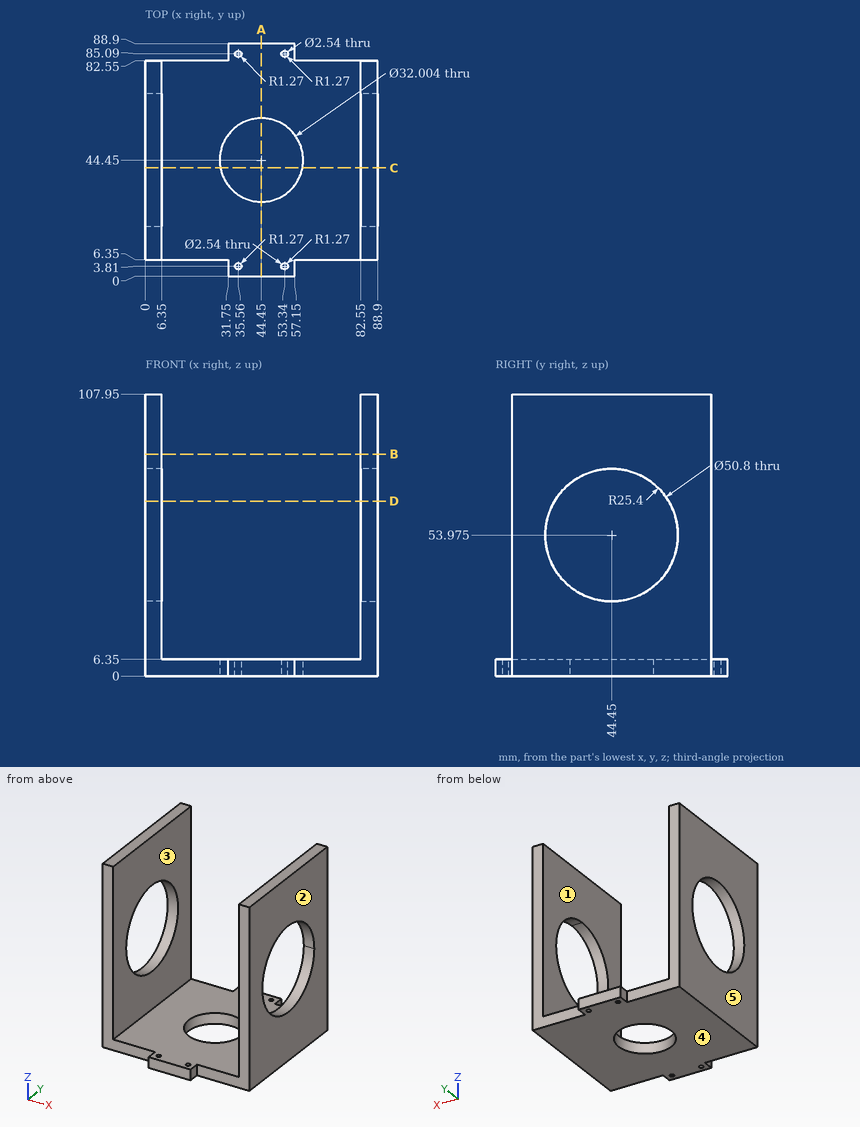
Study the drawing (mm; zero at the part's minimum x, y, z) and answer. A direction names the side the tool comes from. Give positions to 0.01 mm unless a question says otherwise; leave off trailing zeros. Write each loop counter-clockwise with the first axis right and the second up, starting at its lowest first coordinate (ties: lowest second). Pieces come first, ordered by that corner, then holes. Notation, with made-up numbers: (28.25, 79.5) -> (64.25, 79.5) arc R16 ccw to (64.25, 100.5) -> close; hole circle Ø1 at (18, -17). An arc over 180 degrees is marked (long way). Answer in a Markdown table with one row per item.
1) Each of these flat-tipped pins is pushed along its axis until it touches: pin 1 Ø3.5 at (x, y) = (53.34, 85.09) entering from +Z; pin 2 Ø1.9 at (y, z) = (3.5, 4) entering from +X; pin 3 Ø16 at (x, z) = (22, 71.5) entering from +Y; pin 4 Ø1.9 at (y, z) = (4, 3.5) entering from -X. Where does it stop, or does it pass through?
Results list:
| item | result |
|---|---|
| pin 1 | z = 6.35 |
| pin 2 | x = 57.15 |
| pin 3 | through |
| pin 4 | x = 31.75 |
2) Section A-A on x = 44.45 is taken. Give the vertices of the cut face in (y, z).
Results list:
| item | result |
|---|---|
| outline | (0, 0) -> (28.45, 0) -> (28.45, 6.35) -> (0, 6.35) -> close; (60.45, 0) -> (88.9, 0) -> (88.9, 6.35) -> (60.45, 6.35) -> close |
3) Section D-D on z = 67 is taken. Give the vertices of the cut face in (x, y), plus the area to 3 significant figures.
Results list:
| item | result |
|---|---|
| outline | (0, 6.35) -> (6.35, 6.35) -> (6.35, 22.64) -> (0, 22.64) -> close; (0, 66.26) -> (6.35, 66.26) -> (6.35, 82.55) -> (0, 82.55) -> close; (82.55, 6.35) -> (88.9, 6.35) -> (88.9, 22.64) -> (82.55, 22.64) -> close; (82.55, 66.26) -> (88.9, 66.26) -> (88.9, 82.55) -> (82.55, 82.55) -> close |
| area | 414 mm^2 |
4) Section C-C on y = 41.5 is taken. Give the vertices of the cut face in (x, z).
Results list:
| item | result |
|---|---|
| outline | (0, 0) -> (28.72, 0) -> (28.72, 6.35) -> (6.35, 6.35) -> (6.35, 28.75) -> (0, 28.75) -> close; (0, 79.2) -> (6.35, 79.2) -> (6.35, 107.95) -> (0, 107.95) -> close; (60.18, 0) -> (88.9, 0) -> (88.9, 28.75) -> (82.55, 28.75) -> (82.55, 6.35) -> (60.18, 6.35) -> close; (82.55, 79.2) -> (88.9, 79.2) -> (88.9, 107.95) -> (82.55, 107.95) -> close |
5) Determine the mould class of the marked faces 3, 4 and 5 for opening direction X: released by +X, released by -X, zero draft, split by the parting line, or undercut.
Results list:
| item | result |
|---|---|
| face 3 | undercut |
| face 4 | zero draft |
| face 5 | released by -X |
6) Section B-B on z = 85 is taken. Give the vertices of the cut face in (x, y).
Results list:
| item | result |
|---|---|
| outline | (0, 6.35) -> (6.35, 6.35) -> (6.35, 82.55) -> (0, 82.55) -> close; (82.55, 6.35) -> (88.9, 6.35) -> (88.9, 82.55) -> (82.55, 82.55) -> close |
7) Straight lines are drawn through the part: line 1 (X direction, y = 85, z = 4); line 2 (X direction, y = 58.5, z = 9); line 3 (Y direction, x = 53, z = 3). For each, find the intervals that lie inside material, in ascending order. Write a range as [from, to].
Results list:
| item | result |
|---|---|
| line 1 | [31.75, 34.29], [36.83, 52.07], [54.61, 57.15] |
| line 2 | [0, 6.35], [82.55, 88.9] |
| line 3 | [0, 2.59], [5.03, 30.92], [57.98, 83.87], [86.31, 88.9] |
8) A tool of negligible diameter and unlimited length cuts with its end or side. For the marked faces 1 and 2, from which of +Z, -Z, +X, -X, +Y, -Y can it reach the whole face along a straight path? Write none if from no direction.
Results list:
| item | result |
|---|---|
| face 1 | +Z, +Y, -Y |
| face 2 | +Z, -Z, +X, +Y, -Y |
